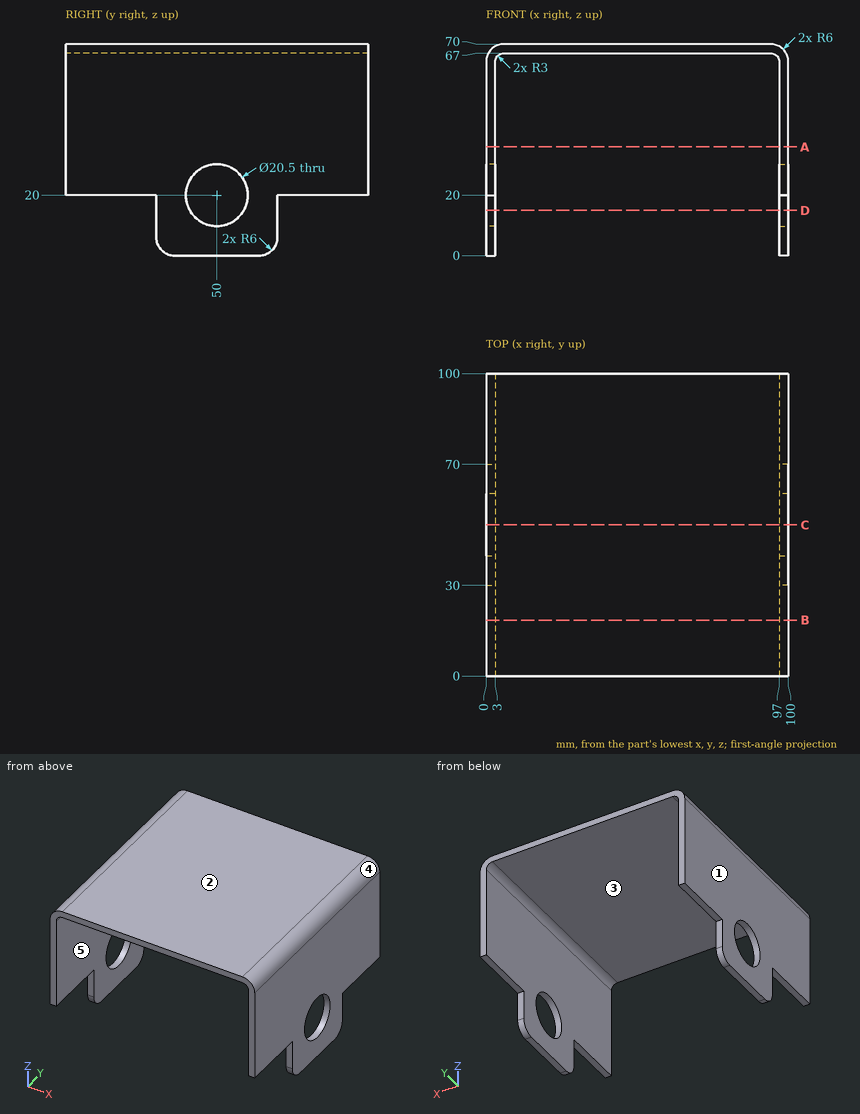
Design review of the part shown in the three views and the two pictorial views. Dimensions are in mm from the part's minimum x, y and z. A direction names the side the tool comes from. Round coordinates to 2 decimals unless told otherwise and drop trailing zeros. Write each loop counter-clockwise with the first axis right and the second up, starting at its lowest first coordinate (ties: lowest second). Pieces come first, ordered by that corner, then holes. Notation, with made-up numbers: (-25.5, -26.5) -> (16.5, -26.5) arc R17 ccw to (16.5, 6.5) -> close; hole circle Ø3 at (25.5, 62). An arc over 180 degrees is marked (long way). Answer as a JSON object with one key per item and string values.
1. The part is to be moulded in two halves that separate along X. For the marked faces 1, 2 and 3, say which applies: pulls with the +X half, pulls with the -X half, needs draft (parallel to the pull), parting line crosses it, or undercut.
Results found:
{"face 1": "pulls with the -X half", "face 2": "needs draft", "face 3": "undercut"}
2. We need section B-B on y = 18.5. State the section outline as (x, z) points.
Results found:
{"outline": "(0, 20) -> (3, 20) -> (3, 64) arc R3 cw to (6, 67) -> (94, 67) arc R3 cw to (97, 64) -> (97, 20) -> (100, 20) -> (100, 64) arc R6 ccw to (94, 70) -> (6, 70) arc R6 ccw to (0, 64) -> close"}
3. Machinability: for the marked faces 4 and 5, which of the approach directions +Z, -Z, +X, -X, +Y, -Y give a long, thin tool a straight path to every point of the face, cutting with its end or side? Answer none if there is none.
Results found:
{"face 4": "+Z, +X, +Y, -Y", "face 5": "-Z, +Y, -Y"}
4. We need section D-D on z = 15. State the section outline as (x, y) points.
Results found:
{"outline": "(0, 30) -> (3, 30) -> (3, 41.05) -> (0, 41.05) -> close; (0, 58.95) -> (3, 58.95) -> (3, 70) -> (0, 70) -> close; (97, 30) -> (100, 30) -> (100, 41.05) -> (97, 41.05) -> close; (97, 58.95) -> (100, 58.95) -> (100, 70) -> (97, 70) -> close"}
5. Clearance check with flat-ended pins moving along their axes: pin 1 (0.9 mm diameter, centred on x = 2, y = 79, fed in from -Z); pin 2 (1.5 mm diameter, centred on x = 2, z = 12.5, fed in from +Y); pin 3 (2.5 mm diameter, centred on x = 1.5, z = 10.5, fed in from -Y). State where each tip first meets the part, or that it passes through.
Results found:
{"pin 1": "stops at z = 20", "pin 2": "stops at y = 70", "pin 3": "stops at y = 30"}
6. We need section A-A on z = 36. State the section outline as (x, y) points.
Results found:
{"outline": "(0, 0) -> (3, 0) -> (3, 100) -> (0, 100) -> close; (97, 0) -> (100, 0) -> (100, 100) -> (97, 100) -> close"}
7. To check wall thickness, follow line 1 along X through (y, z) = (33, 45); line 2 along Z through (x, y) = (55, 71); line 3 along Z through (x, y) = (98, 50). State the ranges of each line that lie inside material, in increasing order.
Results found:
{"line 1": "x = 0 to 3, 97 to 100", "line 2": "z = 67 to 70", "line 3": "z = 0 to 9.75, 30.25 to 68.47"}
8. We need section C-C on y = 50. State the section outline as (x, z) points, and give its area (3 significant figures).
Results found:
{"outline": "(0, 0) -> (3, 0) -> (3, 9.75) -> (0, 9.75) -> close; (0, 30.25) -> (3, 30.25) -> (3, 64) arc R3 cw to (6, 67) -> (94, 67) arc R3 cw to (97, 64) -> (97, 30.25) -> (100, 30.25) -> (100, 64) arc R6 ccw to (94, 70) -> (6, 70) arc R6 ccw to (0, 64) -> close; (97, 0) -> (100, 0) -> (100, 9.75) -> (97, 9.75) -> close", "area": "567 mm^2"}
